```python
from build123d import *

# Parameters (mm, degrees)
SKETCH_1_R      = 1.25
SKETCH_1_R_2    = 1
EXTRUDE_2_DEPTH = 2


with BuildPart() as part:
    # 草圖1 → 填料-伸長2 (new body)
    with BuildSketch(Plane.XY):
        with BuildLine():
            Line((-28.541905067, -9.1179941), (-28.541905067, -34.1179941))
            ThreePointArc((-28.541905067, -34.1179941), (-26.279428563, -40.452876116), (-20.515759037, -43.921253788))
            Line((-20.515759037, -43.921253788), (9.479011757, -49.960601851))
            ThreePointArc((9.479011757, -49.960601851), (16.126000545, -48.308012897), (19.058094933, -42.1179941))
            Line((19.058094933, -42.1179941), (19.058094933, -29.6179941))
            Line((19.058094933, -29.6179941), (17.058094933, -29.6179941))
            ThreePointArc((17.058094933, -29.6179941), (16.350988152, -29.325100881), (16.058094933, -28.6179941))
            Line((16.058094933, -28.6179941), (16.058094933, -26.6179941))
            ThreePointArc((16.058094933, -26.6179941), (16.350988152, -25.910887319), (17.058094933, -25.6179941))
            Line((17.058094933, -25.6179941), (19.058094933, -25.6179941))
            Line((19.058094933, -25.6179941), (19.058094933, -17.6179941))
            Line((19.058094933, -17.6179941), (17.058094933, -17.6179941))
            ThreePointArc((17.058094933, -17.6179941), (16.350988152, -17.325100881), (16.058094933, -16.6179941))
            Line((16.058094933, -16.6179941), (16.058094933, -14.6179941))
            ThreePointArc((16.058094933, -14.6179941), (16.350988152, -13.910887319), (17.058094933, -13.6179941))
            Line((17.058094933, -13.6179941), (19.058094933, -13.6179941))
            Line((19.058094933, -13.6179941), (19.058094933, -1.1179941))
            ThreePointArc((19.058094933, -1.1179941), (16.126000545, 5.072024696), (9.479011757, 6.72461365))
            Line((9.479011757, 6.72461365), (-20.515759037, 0.685265588))
            ThreePointArc((-20.515759037, 0.685265588), (-26.279428563, -2.783112085), (-28.541905067, -9.1179941))
        make_face()
        with Locations((-18.541905067, -9.1179941)):
            Circle(SKETCH_1_R, mode=Mode.SUBTRACT)
        with Locations((15.058094933, -11.6179941)):
            Circle(SKETCH_1_R_2, mode=Mode.SUBTRACT)
        with Locations((15.058094933, -19.6179941)):
            Circle(SKETCH_1_R_2, mode=Mode.SUBTRACT)
        with Locations((15.058094933, -23.6179941)):
            Circle(SKETCH_1_R_2, mode=Mode.SUBTRACT)
        with Locations((-18.541905067, -34.1179941)):
            Circle(SKETCH_1_R, mode=Mode.SUBTRACT)
        with Locations((11.058094933, -1.1179941)):
            Circle(SKETCH_1_R, mode=Mode.SUBTRACT)
        with Locations((15.058094933, -31.6179941)):
            Circle(SKETCH_1_R_2, mode=Mode.SUBTRACT)
        with Locations((11.058094933, -42.1179941)):
            Circle(SKETCH_1_R, mode=Mode.SUBTRACT)
    extrude(amount=EXTRUDE_2_DEPTH)


solid = part.part
```
The listing builds one solid part. Answer for the finished solid, in the listing's coordinates (mm). A direction names the side the tool comes from. Round coordinates to 2 decimals unless told otherwise and drop trailing zeros. Write each loop counter-clockwise with the first axis right and the second up, starting at its lowest first coordinate (ties: lowest second). Pieces come first, ordered by that corner, then holes. Notation, with made-up numbers: (1.25, -9.5) -> (5.25, -9.5) arc R16 ccw to (5.25, 0.5) -> close; hole circle Ø8 at (-10, -22.5). An arc over 180 degrees is marked (long way). Answer as a JSON object with one key per item and string values. Group by question number.
Q1. Straight lines are drawn through the part: line 1 along Y through (x, z) = (10, 0.6); line 2 along Y through (x, z) = (17, 0.75); line 3 along X through (y, z) = (-14.5, 0.65). For each, find the intervals that lie inside material, in ascending order.
Q2. Which of the six approach directions +Z, -Z, +X, -X, +Y, -Y give full straight-line access (tool end or side, diameter ignored) to faces 1 (the face through (18, -13.618, 1)), 2 (the face through (-26.22, -2.71, 0.99))?
Q3. Section C-C (x = -22) is taken. Write down the section's boundary in (y, z).
Q4. Section B-B (y = -38.5) is taken. Write down the section's boundary in (x, z), plus the area to 3 significant figures.
Q5. Determine the mould class of faces 3 (the face through (18, -29.618, 1)), 4 (the face through (-28.542, -21, 1)), 5 (the face through (15.982, -12.001, 0.986)) for opening direction X: pulls with the +X half, pulls with the -X half, needs draft (parallel to the pull), parting line crosses it, or undercut.
Q6. Each of these flat-tipped pins is pushed along its axis until it touches: pin 1 Ø0.6 at (x, z) = (18, 1) entering from -Y; pin 2 Ø0.6 at (y, z) = (-16, 1.5) entering from +X; pin 3 Ø1 at (x, z) = (18.5, 0.5) entering from +Y. Where does it stop, or does it pass through?
Q7. Section A-A (z = 1) is taken. Count the separate pieces of the cut face and the enclosed holes in it, plus the area to 3 significant figures.
Check values:
{
 "1": {"line 1": "-50.05 to -42.78, -41.45 to -1.78, -0.45 to 6.81", "line 2": "-47.47 to -29.62, -25.62 to -17.62, -13.62 to 4.24", "line 3": "-28.54 to 16.07"},
 "2": {"face 1": "+Z, -Z, +X", "face 2": "+Z, -Z, -X, +Y"},
 "3": {"outline": "(-43.5, 0) -> (0.27, 0) -> (0.27, 2) -> (-43.5, 2) -> close"},
 "4": {"outline": "(-27.53, 0) -> (19.06, 0) -> (19.06, 2) -> (-27.53, 2) -> close", "area": "93.2 mm^2"},
 "5": {"face 3": "needs draft", "face 4": "pulls with the -X half", "face 5": "undercut"},
 "6": {"pin 1": "y = -46.58", "pin 2": "x = 16.06", "pin 3": "y = 2.86"},
 "7": {"separate pieces": "1", "enclosed holes": "8", "area": "2,300 mm^2"}
}
